Read the model definition and answer for the solid it produces. Units are mm, in the model's axes. A direction names the side the tool comes from. Coordinates: 2 decimals unless noted, no trailing zeros. Loops run counter-clockwise (first coordinate to the right, second up) from the corner with the lowest first, then second, coordinate; pieces in that order, holes last. Notation, with made-up numbers: (39.5, 17) - (59.5, 17) arc R7 ccw to (59.5, 23) - close; hole circle Ø8 at (8, -37). An arc over 180 degrees is marked (long way). Use one line per item in the form item = value.
from build123d import *

# Parameters (mm, degrees)
F0_W     = 400
F0_H     = 400
F1_DEPTH = 6.35
F2_W     = 400
F2_H     = 400
F2_W_2   = 320
F2_H_2   = 320
F3_DEPTH = 20
F4_W     = 40
F4_H     = 40
F5_DEPTH = 460


# Not quite as in the source:
# - a length typed as a fraction of an inch, garbled in the dataset ("3 / 203.2 mm" for 3/8 in), is restored


with BuildPart() as f1:
    # F0 (on Top) → F1 (new body)
    with BuildSketch(Plane.XY):
        with Locations((200, 200)):
            Rectangle(F0_W, F0_H)
    extrude(amount=F1_DEPTH)

    # F2 (on face) → F3 (join)
    with BuildSketch(Plane.XY.offset(6.35)):
        with Locations((200, 200)):
            Rectangle(F2_W, F2_H)
        with Locations((200, 200)):
            Rectangle(F2_W_2, F2_H_2, mode=Mode.SUBTRACT)
    extrude(amount=F3_DEPTH)

    # F4 (on face) → F5 (join)
    with BuildSketch(Plane.XY.offset(26.35)):
        with Locations((20, 380)):
            Rectangle(F4_W, F4_H)
        with Locations((380, 380)):
            Rectangle(F4_W, F4_H)
        with Locations((380, 20)):
            Rectangle(F4_W, F4_H)
        with Locations((20, 20)):
            Rectangle(F4_W, F4_H)
    extrude(amount=F5_DEPTH)


solid = f1.part
Item 1: The part is cut by section B-B on x = 206.5. Give the vertices of the cut face in (y, z), plus the area to 3 significant figures.
Results below:
outline = (0, 0) - (400, 0) - (400, 26.35) - (360, 26.35) - (360, 6.35) - (40, 6.35) - (40, 26.35) - (0, 26.35) - close
area = 4,140 mm²
Item 2: The part is cut by section A-A on z = 292. Give the vertices of the cut face in (x, y), plus the area to 3 significant figures.
Results below:
outline = (0, 0) - (40, 0) - (40, 40) - (0, 40) - close; (0, 360) - (40, 360) - (40, 400) - (0, 400) - close; (360, 0) - (400, 0) - (400, 40) - (360, 40) - close; (360, 360) - (400, 360) - (400, 400) - (360, 400) - close
area = 6,400 mm²
Item 3: For a pull along Y with two mould halves and no side action, classify faces 1 (the flat face through (36, 0, 188)), 2 (the flat face through (20, 20, 486.35)), 3 (the flat face through (198, 40, 16)), 4 (the flat face through (380, 202, 26.35)) as +Y half, -Y half, draft (parallel to the pull), parting line (faces both ways), or undercut.
Results below:
face_1 = -Y half
face_2 = draft
face_3 = undercut
face_4 = undercut
Item 4: Which of the six approach directions +Z, -Z, +X, -X, +Y, -Y give full straight-line access (tool end or side, diameter ignored) to faces 5 (the flat face through (400, 36, 188)), 6 (the flat face through (380, 360, 253)), 7 (the flat face through (360, 198, 16)), 8 (the flat face through (198, 20, 26.35))?
Results below:
face_5 = +Z, -Z, +X, +Y, -Y
face_6 = +Z, +X, -X
face_7 = +Z
face_8 = +Z, +Y, -Y
Item 5: Each of these flat-tipped pins is pushed along its axis until it touches: P1, Ø2, axis at x = 71.5, y = 251, coming from the +Z side; P2, Ø20, axis at x = 246.5, y = 30, coming from the +Z side. Where does it stop, or does it pass through?
Results below:
P1 = 6.35
P2 = 26.35
Item 6: Find the intervals of material crossed by L1, parallel to Y at x = 369, z = 67.5; L2, parallel to Z at x = 175, y = 124.5, in increasing order.
Results below:
L1 = 0 to 40, 360 to 400
L2 = 0 to 6.35
Item 7: The part is cut by section C-C on y = 375. Give the vertices of the cut face in (x, z), plus the area to 3 significant figures.
Results below:
outline = (0, 0) - (400, 0) - (400, 486.35) - (360, 486.35) - (360, 26.35) - (40, 26.35) - (40, 486.35) - (0, 486.35) - close
area = 47,300 mm²
